```python
from build123d import *

# Parameters (mm, degrees)
F2_DEPTH = 535
F4_DEPTH = 80


with BuildPart() as f2:
    # F1 (on Right) → F2 (new body, symmetric)
    with BuildSketch(Plane.YZ):
        with BuildLine():
            Line((0, 80), (0, 40))
            Line((0, 40), (6, 40))
            Line((6, 40), (6, 63))
            ThreePointArc((6, 63), (8.185015, 68.878434), (13.679108, 71.902541))
            Line((13.679108, 71.902541), (41.587063, 76.043315))
            ThreePointArc((41.587063, 76.043315), (44.028882, 77.387363), (45, 80))
            Line((45, 80), (0, 80))
        make_face()
        with BuildLine():
            Line((6, 40), (0, 40))
            Line((0, 40), (0, 0))
            Line((0, 0), (45, 0))
            ThreePointArc((45, 0), (44.028882, 2.612637), (41.587063, 3.956685))
            Line((41.587063, 3.956685), (13.679108, 8.097459))
            ThreePointArc((13.679108, 8.097459), (8.185015, 11.121566), (6, 17))
            Line((6, 17), (6, 40))
        make_face()
    extrude(amount=F2_DEPTH, both=True)

    # F3 (on face) → F4 (cut, through all)
    with BuildSketch(Plane.XY.offset(80)):
        Polygon((-535, 45), (-535, 0), (-509.019238, 45), align=None)
        Polygon((535, 45), (509.019238, 45), (535, 0), align=None)
    extrude(amount=-F4_DEPTH, mode=Mode.SUBTRACT)


solid = f2.part
```
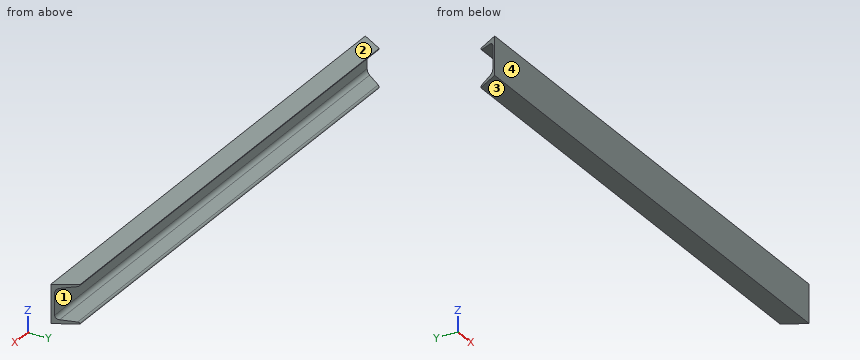
The model under review builds one solid part; all positions refer to its coordinate system, in mm. Face numbers are marked on the shaded views. Give positions to 0.01 mm unless a question says otherwise; leave off trailing zeros. Order: outer loops, then holes, each group sorted by start corner. A loop starts at its lowest first (then second) coordinate and runs counter-clockwise, first axis right, second up. Notation, with made-up numbers: (58, -9.5) - (117, -9.5) arc R20 cw to (117, 0.5) - close; hole circle Ø10 at (79.25, 3). An arc over 180 degrees is marked (long way). Use CSV: the item, a comma, the result in double quotes. Start each with the question number.
Q1. We need section C-C, the plane z = 50. Write out the cut boundary in (x, y), and give its area (3 significant figures).
Q2. We need section B-B, the plane x = 44.5. Write out the cut boundary in (y, z).
Q3. The part is to be moulded in two halves that separate along Z. For the marked faces 1, 2, 3 and 4, say which applies: +Z half, -Z half, draft (parallel to the pull), parting line (faces both ways), or undercut.
Q4. To check wall thickness, follow line 1 along Z through (x, y) = (-384, 14); line 2 along Z through (x, y) = (-240.5, 42); line 3 along Y through (x, z) = (245.5, 32). State the ranges of each line that lie inside material, in increasing order. Write a range as [from, to].
Q5. We need section A-A, the plane y = 21. Write out the cut boundary in (x, z), and give its area (3 significant figures).
Outcome:
1,outline,"(-535, 0) - (535, 0) - (531.54, 6) - (-531.54, 6) - close"
1,area,"6,400 mm^2"
2,outline,"(0, 0) - (45, 0) arc R4 ccw to (41.59, 3.96) - (13.68, 8.1) arc R9 cw to (6, 17) - (6, 63) arc R9 cw to (13.68, 71.9) - (41.59, 76.04) arc R4 ccw to (45, 80) - (0, 80) - close"
3,face 1,"undercut"
3,face 2,"+Z half"
3,face 3,"-Z half"
3,face 4,"draft"
4,line 1,"z = [0, 8.05], [71.95, 80]"
4,line 2,"z = [0, 3.87], [76.13, 80]"
4,line 3,"y = [0, 6]"
5,outline,"(-522.88, 0) - (522.88, 0) - (522.88, 7.01) - (-522.88, 7.01) - close; (-522.88, 72.99) - (522.88, 72.99) - (522.88, 80) - (-522.88, 80) - close"
5,area,"14,700 mm^2"
